Verification items for the finished model (mm, model axes). A direction names the side the tool comes from. Give positions to 0.01 mm unless a question says otherwise; leave off trailing zeros. Write each loop counter-clockwise with the first axis right and the second up, starting at its lowest first coordinate (ties: lowest second). Pieces come first, ordered by that corner, then holes.
from build123d import *

# Parameters (mm, degrees)
CROQUIS1_R                                           = 20
CROQUIS1_R_2                                         = 1
SALIENTE_EXTRUIR1_DEPTH                              = 7
REFRENTADO_PARA_TORNILLO_TAP_N_CON_CABEZ_D           = 3.4
REFRENTADO_PARA_TORNILLO_TAP_N_CON_CABEZ_CSINK_D     = 6.72
REFRENTADO_PARA_TORNILLO_TAP_N_CON_CABEZ_CSINK_ANGLE = 90
TALADRO_DE_MARGEN_PARA_M31_D                         = 3.4
CROQUIS8_R                                           = 5
CORTAR_EXTRUIR1_DEPTH                                = 3


with BuildPart() as part:
    # Croquis1 → Saliente-Extruir1 (new body)
    with BuildSketch(Plane.XY):
        Circle(CROQUIS1_R)
        with Locations((0, 3.6)):
            Circle(CROQUIS1_R_2, mode=Mode.SUBTRACT)
        with Locations((3.117691454, -1.8)):
            Circle(CROQUIS1_R_2, mode=Mode.SUBTRACT)
        with Locations((-3.117691454, -1.8)):
            Circle(CROQUIS1_R_2, mode=Mode.SUBTRACT)
    extrude(amount=SALIENTE_EXTRUIR1_DEPTH)

    # Refrentado para tornillo tapón con cabeza plana de clavija de M31 (through all)
    with Locations(Plane.XY.offset(7)):
        with Locations((0, 15.5), (15.5, 0), (0, -15.5), (-15.5, 0)):
            CounterSinkHole(REFRENTADO_PARA_TORNILLO_TAP_N_CON_CABEZ_D / 2, REFRENTADO_PARA_TORNILLO_TAP_N_CON_CABEZ_CSINK_D / 2, counter_sink_angle=REFRENTADO_PARA_TORNILLO_TAP_N_CON_CABEZ_CSINK_ANGLE)

    # Taladro de margen para M31 (through all)
    with Locations(Plane.XY.offset(7)):
        with Locations((0, 0)):
            Hole(TALADRO_DE_MARGEN_PARA_M31_D / 2)

    # Croquis8 → Cortar-Extruir1 (cut)
    with BuildSketch(Plane(origin=(0, 0, 0), x_dir=(-1, 0, 0), z_dir=(0, 0, -1))):
        Circle(CROQUIS8_R)
    extrude(amount=-CORTAR_EXTRUIR1_DEPTH, mode=Mode.SUBTRACT)


solid = part.part
Item 1: Sectioned sample at C-C on z = 4. State how many separate pieces and enclosed holes the cut face has, then the cut area to 3 significant figures.
Answer key:
separate pieces: 1
enclosed holes: 8
area: 1,200 mm2
Item 2: Release check for a two-part mould opening along X. For faces 1 (the face through (1.08, -4.88, 1.48)), 2 (the face through (-4.336, -19.524, 3.451)), 3 (the face through (0, -4, 7)) record: released by +X, released by -X, zero draft, split by the parting line, or undercut.
Answer key:
face 1: undercut
face 2: split by the parting line
face 3: zero draft
Item 3: Set-up check for faces 4 (the face through (-2, 0, 3)), 5 (the face through (0.37, 13.84, 2.63)): record each of +Z, -Z, +X, -X, +Y, -Y from which the full face is reachable in a straight line by a thin tool's end or side.
Answer key:
face 4: -Z
face 5: +Z, -Z
Item 4: Sectioned sample at B-B on y = 0. Record the cut outline in (x, z), then the cut area to 3 significant figures.
Answer key:
outline: (-20, 0) - (-17.2, 0) - (-17.2, 5.34) - (-18.86, 7) - (-20, 7) - close; (-13.8, 0) - (-5, 0) - (-5, 3) - (-1.7, 3) - (-1.7, 7) - (-12.14, 7) - (-13.8, 5.34) - close; (1.7, 3) - (5, 3) - (5, 0) - (13.8, 0) - (13.8, 5.34) - (12.14, 7) - (1.7, 7) - close; (17.2, 0) - (20, 0) - (20, 7) - (18.86, 7) - (17.2, 5.34) - close
area: 183 mm2
Item 5: Depth check by flat-ended pin: pin 1 (4 mm diameter, centred on x = 0, y = 0, fed in from -Z); pin 2 (4 mm diameter, centred on y = 6.5, z = 2.5, fed in from -X); pin 3 (3 mm diameter, centred on y = -5, z = 4.5, fed in from +X); pin 4 (1.2 mm diameter, centred on x = 0, y = 3.6, fed in from -Z). Enter the tip coordinate at first touch or a pass-through.
Answer key:
pin 1: stops at z = 3
pin 2: stops at x = -19.49
pin 3: stops at x = 19.69
pin 4: passes through
Item 6: Scan lines: line 1 along X through (y, z) = (-1.8, 4.15); line 2 along X through (y, z) = (3.6, 4.45); line 3 along X through (y, z) = (15, 5). Record each from-to range of solid material in increasing order.
Answer key:
line 1: x = -19.92 to -4.12, -2.12 to 2.12, 4.12 to 19.92
line 2: x = -19.67 to -1, 1 to 19.67
line 3: x = -13.23 to -1.62, 1.62 to 13.23
Item 7: Sectioned sample at A-A on x = 0. Record the cut outline in (y, z), then the cut area to 3 significant figures.
Answer key:
outline: (-20, 0) - (-17.2, 0) - (-17.2, 5.34) - (-18.86, 7) - (-20, 7) - close; (-13.8, 0) - (-5, 0) - (-5, 3) - (-1.7, 3) - (-1.7, 7) - (-12.14, 7) - (-13.8, 5.34) - close; (1.7, 3) - (2.6, 3) - (2.6, 7) - (1.7, 7) - close; (4.6, 3) - (5, 3) - (5, 0) - (13.8, 0) - (13.8, 5.34) - (12.14, 7) - (4.6, 7) - close; (17.2, 0) - (20, 0) - (20, 7) - (18.86, 7) - (17.2, 5.34) - close
area: 175 mm2
Item 8: Sectioned sample at D-D on y = -15.5. Record the cut outline in (x, z).
Answer key:
outline: (-12.64, 0) - (-1.7, 0) - (-1.7, 5.34) - (-3.36, 7) - (-12.64, 7) - close; (1.7, 0) - (12.64, 0) - (12.64, 7) - (3.36, 7) - (1.7, 5.34) - close
